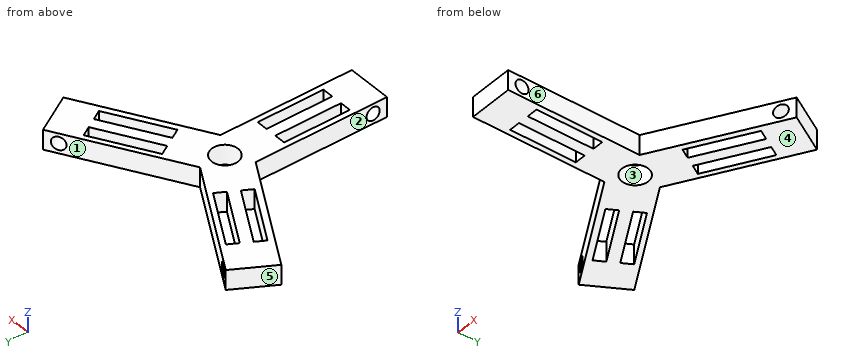
from build123d import *

# Parameters (mm, degrees)
SKETCH2_R           = 60
BOSS_EXTRUDE1_DEPTH = 90
SKETCH4_W           = 50
SKETCH4_H           = 300
CUT_EXTRUDE1_DEPTH  = 90
CIRPATTERN1_COUNT   = 3
SKETCH7_R           = 30
CUT_EXTRUDE2_DEPTH  = 770.615242271
CIRPATTERN2_COUNT   = 3


with BuildPart() as part:
    # Sketch2 → Boss-Extrude1 (new body)
    with BuildSketch(Plane.XY):
        Polygon((-100, -60), (-100, -660), (100, -660), (100, -60), (619.615242271, 240), (519.615242271, 413.205080757), (0, 113.205080757), (-519.615242271, 413.205080757), (-619.615242271, 240), align=None)
        Circle(SKETCH2_R, mode=Mode.SUBTRACT)
    extrude(amount=BOSS_EXTRUDE1_DEPTH)

    # Sketch4 → Cut-Extrude1 (cut)
    with BuildSketch(Plane.XY.offset(90)):
        with Locations((-50, -360.309938914)):
            Rectangle(SKETCH4_W, SKETCH4_H)
        with Locations((50, -360.309938914)):
            Rectangle(SKETCH4_W, SKETCH4_H)
    cut_extrude1 = extrude(amount=-CUT_EXTRUDE1_DEPTH, mode=Mode.SUBTRACT)

    # CirPattern1: Cut-Extrude1 ×3 about axis
    cirpattern1_axis = Axis((0, 0, 0), (0, 0, 1))
    for i in range(1, CIRPATTERN1_COUNT):
        add(cut_extrude1.rotate(cirpattern1_axis, i * 360 / CIRPATTERN1_COUNT), mode=Mode.SUBTRACT)

    # Sketch7 → Cut-Extrude2 (cut, through all)
    with BuildSketch(Plane(origin=(-50.980762114, -88.301270189, 0), x_dir=(0.866025404, -0.5, 0), z_dir=(-0.5, -0.866025404, 0))):
        with Locations((-596.602540378, 45)):
            Circle(SKETCH7_R)
    cut_extrude2 = extrude(amount=-CUT_EXTRUDE2_DEPTH, mode=Mode.SUBTRACT)

    # CirPattern2: Cut-Extrude2 ×3 about axis
    cirpattern2_axis = Axis((0, 0, 0), (0, 0, 1))
    for i in range(1, CIRPATTERN2_COUNT):
        add(cut_extrude2.rotate(cirpattern2_axis, i * 360 / CIRPATTERN2_COUNT), mode=Mode.SUBTRACT)


solid = part.part
Build history of the part. All positions in model axes, mm. Face numbers are marked on the shaded views. A direction names the side the tool comes from. Round coordinates to 2 decimals unless told otherwise and drop trailing zeros. Write each loop counter-clockwise with the first axis right and the second up, starting at its lowest first coordinate (ties: lowest second). Pieces come first, ordered by that corner, then holes. Notation, with made-up numbers: M 58,-14 L 109,-14 A15 cw 109,-9 Z; hole C 55,86 d7. An arc over 180 degrees is marked long. Answer in a Markdown table with one row per item.
1. Saw through at A-A (y = -447). List the corners of the cut face in (x, z), and give its area (3 significant figures).
Geometry check:
| item | result |
|---|---|
| outline | M -100,0 L -75,0 L -75,90 L -100,90 Z; M -25,0 L 25,0 L 25,90 L -25,90 Z; M 75,0 L 100,0 L 100,90 L 75,90 Z |
| area | 9,000 mm2 |
2. Mould opens along X. For the marked faces 1, 2, 3 and 4 say: +X half, -X half, draft (parallel to the pull), parting line (faces both ways), or undercut.
Geometry check:
| item | result |
|---|---|
| face 1 | undercut |
| face 2 | -X half |
| face 3 | undercut |
| face 4 | draft |
3. Flat gauge pins, fed straight in: P1, Ø1.5, axis at y = 272, z = 31.5, coming from the -X side; P2, Ø25, axis at x = -39.5, z = 60.5, coming from the +Y side; P3, Ø4, axis at y = 229, z = 32, coming from the +X side. Where does each tip first touch, or does it go through?
Geometry check:
| item | result |
|---|---|
| P1 | x = -601.57 |
| P2 | y = 143.23 |
| P3 | x = 604.03 |
4. Saw through at C-C (y = 0). List the corners of the cut face in (x, z), and give its area (3 significant figures).
Geometry check:
| item | result |
|---|---|
| outline | M -203.92,0 L -60,0 L -60,90 L -203.92,90 Z; M 60,0 L 203.92,0 L 203.92,90 L 60,90 Z |
| area | 25,900 mm2 |
5. Which spindle directions (+Z, -Z, +X, -X, +Y, -Y) get a long thin tool onto all of the face, cutting with end or side? Do the marked faces 5 and 6. Say none if no direction does.
Geometry check:
| item | result |
|---|---|
| face 5 | +Z, -Z, -X, +Y |
| face 6 | +Z, -Z, +X, -Y |
6. Saw through at D-D (z = 29.5). State how many separate pieces and enclosed holes the cut face has, and give its area (3 significant figures).
Geometry check:
| item | result |
|---|---|
| separate pieces | 4 |
| enclosed holes | 7 |
| area | 245,000 mm2 |
7. Probe L1, parallel to X at y = -454, z = 61; L2, parallel to Y at x = 0, z = 47; L3, parallel to Y at x = 0, z = 19. List the from-to ranges inside material, lowest first. Write a range as [from, to].
Geometry check:
| item | result |
|---|---|
| L1 | [-100, -75], [-25, 25], [75, 100] |
| L2 | [-660, -626.54], [-566.67, -60], [60, 113.21] |
| L3 | [-660, -611.57], [-581.64, -60], [60, 113.21] |
8. Saw through at B-B (x = -361.5). List the corners of the cut face in (y, z).
Geometry check:
| item | result |
|---|---|
| outline | M 90.98,0 L 122.11,0 L 122.11,90 L 90.98,90 Z; M 179.84,0 L 237.58,0 L 237.58,90 L 179.84,90 Z; M 295.31,0 L 321.92,0 L 321.92,90 L 295.31,90 Z |
